Check sheet for the drawn part. Datum: minimum x, y, z corner. Units: mm. A direction names the side the tool comes from. Round coordinates to 2 decimals unless told otherwise and drop trailing zeros. Write each loop counter-clockwise with the first axis right and the second up, starting at its lowest first coordinate (ties: lowest second). Pieces come first, ordered by that corner, then holes. Notation, with made-up numbers: M 77,13.25 L 97,13.25 A17 cw 97,18.25 Z; hole C -23,25.25 d4. An arc over 180 degrees is marked long. Use a Markdown table: item, result.
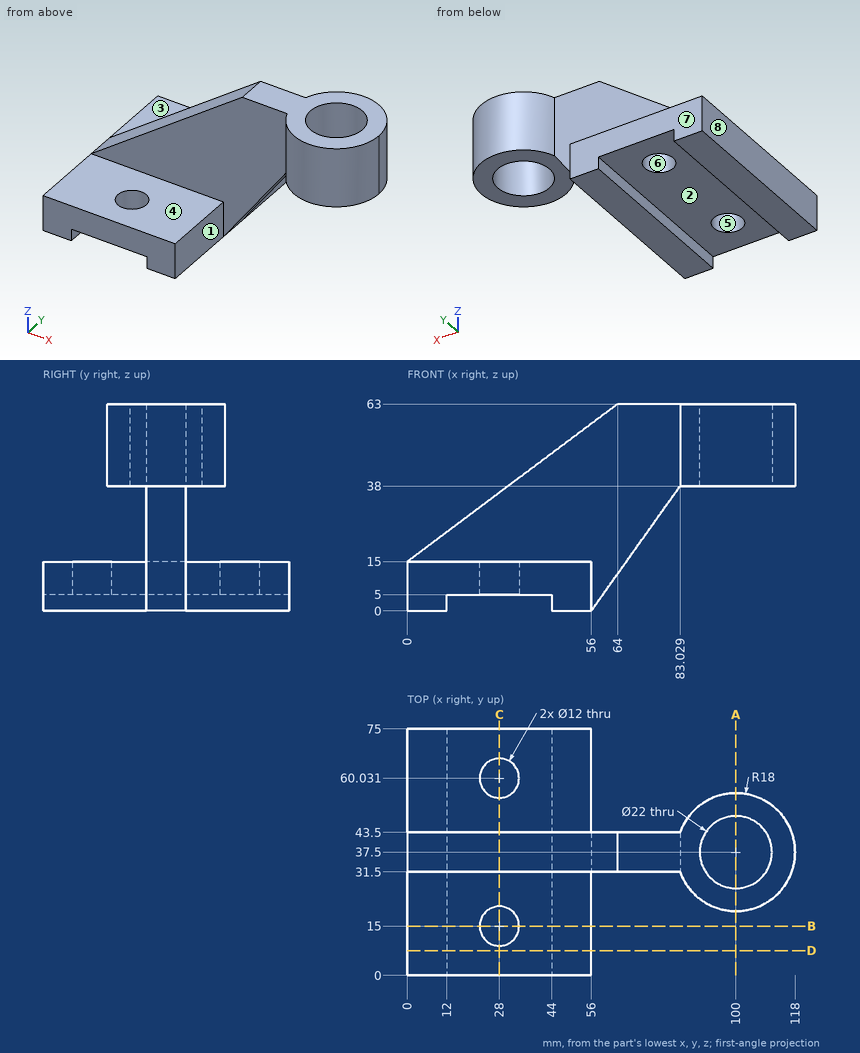
Item 1: Access from +Z, -Z, +X, -X, +Y, -Y to the whole of each face (thin tool, end or side, straight path). Record for the marked faces 1, 2, 3 and 4.
Outcome:
| item | result |
|---|---|
| face 1 | +Z, -Z, +X, -Y |
| face 2 | -Z, +Y, -Y |
| face 3 | +Z, +X, -X, +Y |
| face 4 | +Z, +X, -X, -Y |
Item 2: Material ranges on line 1 along Y through (x, z) = (28, 9.75); line 2 along Y through (x, z) = (100, 52); line 3 along Y through (x, z) = (68, 37), recorded low to high. Write a range as from..to.
Outcome:
| item | result |
|---|---|
| line 1 | y = 0..9, 21..54.03, 66.03..75 |
| line 2 | y = 19.5..26.5, 48.5..55.5 |
| line 3 | y = 31.5..43.5 |
Item 3: Go/stop test with flat-tipped pins: pin 1 (19 mm diameter, centred on x = 23, z = 44, fed in from -Y); pin 2 (12 mm diameter, centred on x = 27.5, z = 31, fed in from +Y); pin 3 (15.5 mm diameter, centred on x = 28, y = 60.03, fed in from -Z); pin 4 (1.5 mm diameter, centred on x = 44, y = 44, fed in from -Z). Record where each tip stops, or that it passes through.
Outcome:
| item | result |
|---|---|
| pin 1 | stops at y = 31.5 |
| pin 2 | stops at y = 43.5 |
| pin 3 | stops at z = 5 |
| pin 4 | stops at z = 0 |
Item 4: Cross-section at D-D, the plane y = 7.5. Record the cut outline in (x, z), and give its area (3 significant figures).
Outcome:
| item | result |
|---|---|
| outline | M 0,0 L 12,0 L 12,5 L 44,5 L 44,0 L 56,0 L 56,15 L 0,15 Z |
| area | 680 mm2 |
Item 5: Cross-section at B-B, the plane y = 15. Record the cut outline in (x, z).
Outcome:
| item | result |
|---|---|
| outline | M 0,0 L 12,0 L 12,5 L 22,5 L 22,15 L 0,15 Z; M 34,5 L 44,5 L 44,0 L 56,0 L 56,15 L 34,15 Z |
Item 6: Mould release check, pull along Y, two halves, no side actions. Record for the marked faces 5, 6, 7 and 8: +Y half, -Y half, draft (parallel to the pull), parting line (faces both ways), or undercut.
Outcome:
| item | result |
|---|---|
| face 5 | undercut |
| face 6 | undercut |
| face 7 | +Y half |
| face 8 | draft |
Item 7: Cross-section at C-C, the plane x = 28. Record the cut outline in (y, z), and give its area (3 significant figures).
Outcome:
| item | result |
|---|---|
| outline | M 0,5 L 9,5 L 9,15 L 0,15 Z; M 21,5 L 54.03,5 L 54.03,15 L 43.5,15 L 43.5,36 L 31.5,36 L 31.5,15 L 21,15 Z; M 66.03,5 L 75,5 L 75,15 L 66.03,15 Z |
| area | 762 mm2 |
Item 8: Cross-section at A-A, the plane x = 100. Record the cut outline in (y, z).
Outcome:
| item | result |
|---|---|
| outline | M 19.5,38 L 26.5,38 L 26.5,63 L 19.5,63 Z; M 48.5,38 L 55.5,38 L 55.5,63 L 48.5,63 Z |
